Geometry: final body of the model. Coordinates: model frame, mm. Round coordinates to 2 decimals unless told otherwise and drop trailing zeros. Loops run counter-clockwise (first coordinate to the right, second up) from the corner with the lowest first, then second, coordinate; pieces in that order, holes last. Notation, with made-up numbers: M 21.5,82 L 38.5,82 A33 ccw 38.5,119 Z; hole C 11.5,37.25 d8. An arc over 180 degrees is marked long. Answer as a JSON object with one key per item and string values.
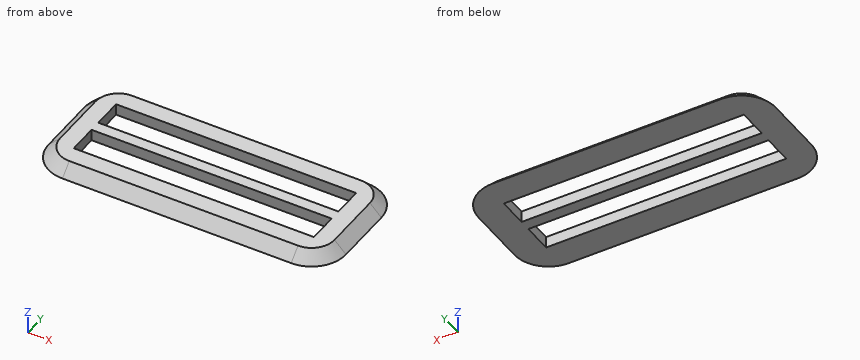
from build123d import *

# Parameters (mm, degrees)
F0_W     = 26
F0_H     = 11.2
F0_W_2   = 21
F0_H_2   = 2.6
F1_DEPTH = 1
F2_R     = 3
F3_SIZE  = 0.99999


# Not quite as in the source:
# - a fillet or chamfer is up to 0.001 mm smaller than in the source, because OpenCascade refuses the exact size


with BuildPart() as f1:
    # F0 (on Top) → F1 (new body)
    with BuildSketch(Plane.XY):
        Rectangle(F0_W, F0_H)
        with Locations((0, -1.8)):
            Rectangle(F0_W_2, F0_H_2, mode=Mode.SUBTRACT)
        with Locations((0, 1.8)):
            Rectangle(F0_W_2, F0_H_2, mode=Mode.SUBTRACT)
    extrude(amount=F1_DEPTH)

    # F2
    f2_edges = [f1.edges().sort_by_distance(p)[0] for p in [
        (-13, 5.6, 0.5),
        (-13, -5.6, 0.5),
        (13, -5.6, 0.5),
        (13, 5.6, 0.5),
    ]]
    fillet(f2_edges, radius=F2_R)

    # F3 (size 1 in the source; OpenCascade refuses exactly that, so slightly less here)
    f3_edges = [f1.edges().sort_by_distance(p)[0] for p in [
        (-12.12132, -4.72132, 1),
    ]]
    chamfer(f3_edges, length=F3_SIZE)


solid = f1.part
1) Section query A-A (x = 2.25). Count the separate pieces of the cut face and the enclosed holes in it, and give its area (3 significant figures).
Results:
{"separate pieces": "3", "enclosed holes": "0", "area": "5.00 mm2"}
2) Section query C-C (z = 0.75). Return the cut outline in (x, y), and give its area (3 significant figures).
Results:
{"outline": "M -12.25,-2.6 A2.25 ccw -10,-4.85 L 10,-4.85 A2.25 ccw 12.25,-2.6 L 12.25,2.6 A2.25 ccw 10,4.85 L -10,4.85 A2.25 ccw -12.25,2.6 Z; hole M -10.5,-3.1 L 10.5,-3.1 L 10.5,-0.5 L -10.5,-0.5 Z; hole M -10.5,0.5 L 10.5,0.5 L 10.5,3.1 L -10.5,3.1 Z", "area": "124 mm2"}
3) Pin query (flat end, axial travel): P1, Ø0.5, axis at x = -3, z = 0.5, coming from the +Y side; P2, Ø0.5, axis at x = -4, z = 0.5, coming from the -Y side. Return the tip coordinate at first contact, or that it passes through.
Results:
{"P1": "y = 5.35", "P2": "y = -5.35"}
4) Ray query, line 1 (Y direction, x = 5.25, z = 0.4); line 2 (Y direction, x = -7.5, z = 0.7); line 3 (X direction, y = -2.75, z = 0.2). Return the intervals inside material, ascending.
Results:
{"line 1": "-5.2 to -3.1, -0.5 to 0.5, 3.1 to 5.2", "line 2": "-4.9 to -3.1, -0.5 to 0.5, 3.1 to 4.9", "line 3": "-12.8 to -10.5, 10.5 to 12.8"}
